Check sheet for the modelled part. Datum: model origin and axes. Units: mm. Face numbers are marked on the shaded views. A direction names the side the tool comes from. Give positions to 0.01 mm unless a question says otherwise; leave off trailing zeros. Write each loop counter-clockwise with the first axis right and the second up, starting at its lowest first coordinate (ties: lowest second). Pieces come first, ordered by that corner, then holes. Notation, with made-up numbers: (34.5, -4) -> (71.5, -4) arc R21 ccw to (71.5, 35) -> close; hole circle Ø1 at (42.25, 51.25). An arc over 180 degrees is marked (long way). Write each question's results on one line, items separated by ' | '. Start each with the question number.
```python
from build123d import *

# Parameters (mm, degrees)
F0_W      = 159.493204
F0_H      = 92.830694
F1_DEPTH  = 25.4
F2_T      = -2.54
F1_FACE_W = 92.830694
F1_FACE_H = 25.4
F3_DEPTH  = 2.54


with BuildPart() as f1:
    # F0 (on Top) → F1 (new body)
    with BuildSketch(Plane.XY):
        with Locations((-0.945693, -4.521475)):
            Rectangle(F0_W, F0_H)
    extrude(amount=F1_DEPTH)

    # F2
    f2_openings = [f1.faces().sort_by_distance(p)[0] for p in [
        (-0.945693, -4.521475, 25.4),
    ]]
    offset(amount=F2_T, openings=f2_openings)

    # F1_face (on face) → F3 (cut)
    with BuildSketch(Plane(origin=(-80.692295, -4.521475, 12.7), x_dir=(0, -1, 0), z_dir=(-1, 0, 0))):
        Rectangle(F1_FACE_W, F1_FACE_H)
    extrude(amount=-F3_DEPTH, mode=Mode.SUBTRACT)


solid = f1.part
```
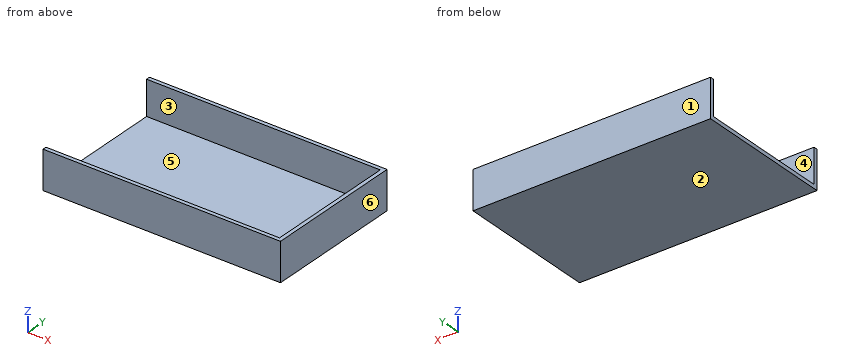
Item 1: Depth check by flat-ended pin: pin 1 Ø1.5 at (y, z) = (3, 22) entering from -X. Enter the tip coordinate at first touch or a pass-through.
Item 2: Thickness scan on probe 1 along Y at (x, z) = (-60, 5.25); probe 2 along Z at (x, y) = (5, -29); probe 3 along X at (y, z) = (15, 13.25). Record the ranges inside material, lowest first. Write a range as from..to.
Item 3: Mould release check, pull along Y, two halves, no side actions. Record for the marked faces 1, 2, 3 and 4: pulls with the +Y half, pulls with the -Y half, needs draft (parallel to the pull), parting line crosses it, or undercut.
Item 4: Section check C-C on y = -20. Record the boundary of the cut face in (x, z), then the cut area to 3 significant figures.
Item 5: Section check A-A on z = 19. Record the boundary of the cut face in (x, y).
Item 6: Set-up check for the marked faces 5 and 6: record each of +Z, -Z, +X, -X, +Y, -Y from which the full face is reachable in a straight line by a thin tool's end or side.
Item 7: Section check B-B on x = 50. Record the boundary of the cut face in (y, z).
Check sheet entries:
1) pin 1: stops at x = 76.26
2) probe 1: y = -50.94..-48.4, 39.35..41.89 | probe 2: z = 0..2.54 | probe 3: x = 76.26..78.8
3) face 1: pulls with the +Y half | face 2: needs draft | face 3: undercut | face 4: undercut
4) outline: (-78.15, 0) -> (78.8, 0) -> (78.8, 25.4) -> (76.26, 25.4) -> (76.26, 2.54) -> (-78.15, 2.54) -> close | area: 457 mm^2
5) outline: (-78.15, -50.94) -> (78.8, -50.94) -> (78.8, 41.89) -> (-78.15, 41.89) -> (-78.15, 39.35) -> (76.26, 39.35) -> (76.26, -48.4) -> (-78.15, -48.4) -> close
6) face 5: +Z, -X | face 6: +Z, -Z, +X, +Y, -Y
7) outline: (-50.94, 0) -> (41.89, 0) -> (41.89, 25.4) -> (39.35, 25.4) -> (39.35, 2.54) -> (-48.4, 2.54) -> (-48.4, 25.4) -> (-50.94, 25.4) -> close
